Geometry: final body of the model. Coordinates: model frame, mm. Face numbers are marked on the shaded views. Give positions to 0.01 mm unless a question says otherwise; leave off trailing zeros. Order: outer loops, then holes, each group sorted by start corner. A loop starts at its lowest first (then second) coordinate and runs counter-clockwise, first axis right, second up. Notation, with made-up numbers: (47, 68) -> (66, 68) arc R32 ccw to (66, 96) -> close; hole circle Ø6 at (-18.5, 47). An arc over 180 degrees is marked (long way). One line per question, with ' | ' between items.
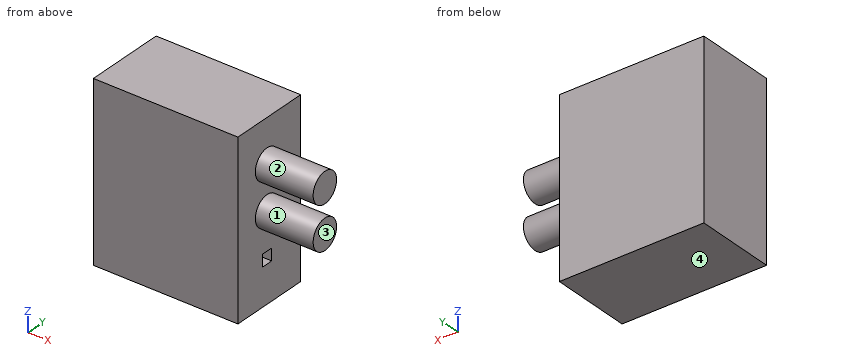
from build123d import *

# Parameters (mm, degrees)
F0_W     = 39.6875
F0_H     = 47.625
F1_DEPTH = 22.225
F2_R     = 4.1548957558
F3_DEPTH = 15.875
F2_W     = 3.302
F2_H     = 3.302
F4_DEPTH = 12.7


# Not quite as in the source:
# - a length typed as a fraction of an inch, garbled in the dataset ("3 / 203.2 mm" for 3/8 in), is restored


with BuildPart() as f1:
    # F0 (on Front) → F1 (new body)
    with BuildSketch(Plane.XZ):
        with Locations((-3.6287705289, -8.4221055731)):
            Rectangle(F0_W, F0_H)
    extrude(amount=F1_DEPTH)

    # F2 (on face) → F3 (join)
    with BuildSketch(Plane.YZ.offset(16.2149794711)):
        with Locations((-11.90625, 3.4968444269)):
            Circle(F2_R)
        with Locations((-11.90625, -8.4157555731)):
            Circle(F2_R)
    extrude(amount=F3_DEPTH)

    # F2 (on face) → F4 (cut)
    with BuildSketch(Plane.YZ.offset(16.2149794711)):
        with Locations((-11.90625, -20.3283555731)):
            Rectangle(F2_W, F2_H)
    extrude(amount=-F4_DEPTH, mode=Mode.SUBTRACT)


solid = f1.part
1) Pull-direction query (Z, two-part tool) for the marked faces 1, 2, 3 and 4; classes: +Z half, -Z half, draft (parallel to the pull), parting line (faces both ways), or undercut.
Check result:
face 1: undercut | face 2: undercut | face 3: draft | face 4: -Z half
2) Material intervals for probe 1 along X at (y, z) = (-14.75, -17); probe 2 along Z at (x, y) = (20, -14.25); probe 3 along X at (y, z) = (-10.5, -19), sorted ascending. Write a range as from..to.
Check result:
probe 1: x = -23.47..16.21 | probe 2: z = -11.85..-4.99, 0.07..6.93 | probe 3: x = -23.47..3.51
3) Section C-C on x = 23. Return loops of the section in (y, z), plus the area to 3 significant figures.
Check result:
outline: circle Ø8.31 at (-11.91, -8.42); circle Ø8.31 at (-11.91, 3.5) | area: 108 mm^2
4) Section A-A on z = -11. Return loops of the section in (x, y) (3 decimals), plus the area to 3 significant figures.
Check result:
outline: (-23.473, -22.225) -> (16.215, -22.225) -> (16.215, -15.16) -> (32.09, -15.16) -> (32.09, -8.653) -> (16.215, -8.653) -> (16.215, 0) -> (-23.473, 0) -> close | area: 985 mm^2
5) Section B-B on y = -12.75. Return loops of the section in (x, z).
Check result:
outline: (-23.47, -32.23) -> (16.21, -32.23) -> (16.21, -21.98) -> (3.51, -21.98) -> (3.51, -18.68) -> (16.21, -18.68) -> (16.21, -12.48) -> (32.09, -12.48) -> (32.09, -4.35) -> (16.21, -4.35) -> (16.21, -0.57) -> (32.09, -0.57) -> (32.09, 7.57) -> (16.21, 7.57) -> (16.21, 15.39) -> (-23.47, 15.39) -> close
6) Section D-D on y = -8.5. Return loops of the section in (x, z).
Check result:
outline: (-23.47, -32.23) -> (16.21, -32.23) -> (16.21, -10.79) -> (32.09, -10.79) -> (32.09, -6.04) -> (16.21, -6.04) -> (16.21, 1.12) -> (32.09, 1.12) -> (32.09, 5.88) -> (16.21, 5.88) -> (16.21, 15.39) -> (-23.47, 15.39) -> close
7) Contact query for flat-ended pins moving along their axis: pin 1 Ø1 at (y, z) = (-9, -22) entering from +X (3 decimals); pin 2 Ø3 at (x, y) = (20.5, -16.5) entering from -Z; pin 3 Ø2 at (x, z) = (24, 1) entering from -Y. Output: stop coordinate, or through.
Check result:
pin 1: stops at x = 16.215 | pin 2: stops at z = -11.19 | pin 3: stops at y = -15.78
